For this review, take the finished solid that the model builds, in its own axes (mm). A direction names the side the tool comes from. Coordinates: 2 decimals unless noted, no trailing zeros. Order: outer loops, then holes, each group sorted by start corner. A loop starts at its lowest first (then second) coordinate and runs counter-clockwise, first axis right, second up. Notation, with made-up numbers: (-35.75, 63.25) -> (22.25, 63.25) arc R24 ccw to (22.25, 76.25) -> close; hole circle Ø4 at (10.25, 78.25). An arc over 180 degrees is marked (long way). Return JSON: item names as keys, results as strings. Group by question number.
Item 1: Draft analysis for pull direction Z (two halves, no side actions). For faces 4 (the cylindrical face through (-10.161, -4.213, -40.439)), 5 (the cylindrical face through (0.53, -11.99, -42.9)), 6 (the conical face through (1.627, 5.166, 32.753)), state which applies: +Z half, -Z half, draft (parallel to the pull), parting line (faces both ways), or undercut.
Item 2: For line 1 along Z through (x, y) = (10.25, 6); line 2 along X through (y, z) = (0, 2); line 3 along X through (y, z) = (0, -37.6), list the stretches that pass through material, from the lowest coordinate up.
Item 3: Insertion check: pin 1 (1 mm diameter, centred on x = -8.5, z = -33, fed in from +Y); pin 2 (6 mm diameter, centred on x = 9.5, z = 12.5, fed in from -Y); pin 3 (13 mm diameter, centred on x = 0, y = 0, fed in from -Z). Each pin has a flat end and moves straight along its axis. Give the tip position at first contact, or say it passes through.
Item 4: Take a section at A-A (z = 11). Write out the cut boundary in (x, y).
Item 5: Machinability: for faces 1 (the cylindrical face through (-4.213, 10.161, -7.999)), 2 (the flat face through (11, 2, -51.918)), 3 (the flat face through (-10, 5, -41.918)), which of the approach directions +Z, -Z, +X, -X, +Y, -Y give a long, thin tool a straight path to every point of the face, cutting with its end or side? Answer none if there is none.
Item 6: Take a section at B-B (z = 34.5). Write out the cut boundary in (x, y), then the cut area to 3 significant figures.
```python
from build123d import *

# Parameters (mm, degrees)
ESQUISSE2_R             = 11
ENL_V_MAT_EXTRU_1_DEPTH = 15
CONG_1_R                = 5
CHANFREIN1_SIZE         = 1
CHANFREIN1_SIZE2        = 0.577350269


with BuildPart() as part:
    # Esquisse1 → Révolution1 (revolve)
    with BuildSketch(Plane(origin=(0, 0, 0), x_dir=(0, 0, -1), z_dir=(1, 0, 0))):
        Polygon((36.918161096, 11), (36.918161096, 9), (51.918161096, 9), (51.918161096, 14.5), (-51.918161096, 14.5), (-51.918161096, 5.5), (-37.804270768, 2.5), (-23.081838904, 11), align=None)
    revolve(axis=Axis((0, 0, 51.918161096), (0, 0, -1)))

    # Esquisse2 → Enlèv. mat.-Extru.1 (cut)
    with BuildSketch(Plane(origin=(0, 0, -51.918161096), x_dir=(-1, 0, 0), z_dir=(0, 0, -1))):
        Circle(ESQUISSE2_R)
    extrude(amount=-ENL_V_MAT_EXTRU_1_DEPTH, mode=Mode.SUBTRACT)

    # Esquisse3 → Enlèvement de matière-Révolution1 (revolve, cut)
    with BuildSketch(Plane(origin=(0, 0, 0), x_dir=(0, 0, -1), z_dir=(1, 0, 0))):
        Polygon((48.918161096, 11), (48.918161096, 12), (46.918161096, 12), (46.918161096, 11), (43.918161096, 11), (43.918161096, 12), (41.918161096, 12), (41.918161096, 11), (38.918161096, 11), (38.918161096, 12), (36.918161096, 12), (36.918161096, 11), (36.918161096, 0), (51.918161096, 0), (51.918161096, 11), align=None)
    revolve(axis=Axis((0, 0, 0), (0, 0, -1)), mode=Mode.SUBTRACT)

    # Congé1
    cong_1_edges = [part.edges().sort_by_distance(p)[0] for p in [
        (0, -11, 23.081838904),
        (0, -2.5, 37.804270768),
    ]]
    fillet(cong_1_edges, radius=CONG_1_R)

    # Chanfrein1
    chanfrein1_edges = [part.edges().sort_by_distance(p)[0] for p in [
        (0, -14.5, 51.918161096),
    ]]
    chanfrein1_side = [part.faces().sort_by_distance(p)[0] for p in [
        (0, -14.5, 0),
    ]]
    chamfer(chanfrein1_edges, length=CHANFREIN1_SIZE, length2=CHANFREIN1_SIZE2, reference=chanfrein1_side[0])


solid = part.part
```
Findings below:
{
 "1": {"face 4": "draft", "face 5": "undercut", "face 6": "-Z half"},
 "2": {"line 1": "z = -51.92 to -48.92, -46.92 to -43.92, -41.92 to -38.92, -36.92 to 51.92", "line 2": "x = -14.5 to -11, 11 to 14.5", "line 3": "x = -14.5 to -12, 12 to 14.5"},
 "3": {"pin 1": "stops at y = 12.09", "pin 2": "stops at y = -12.96", "pin 3": "stops at z = 30.88"},
 "4": {"outline": "circle Ø29 at (0, 0); hole circle Ø22 at (0, 0)"},
 "5": {"face 1": "-Z", "face 2": "-Z, +X, -X, +Y, -Y", "face 3": "none"},
 "6": {"outline": "circle Ø29 at (0, 0); hole circle Ø8.82 at (0, 0)", "area": "599 mm2"}
}
